```python
from build123d import *

# Parameters (mm, degrees)
F0_R          = 3
F0_R_2        = 2.5
F1_DEPTH      = 150
F2_R          = 2
F3_R          = 7
F6_DEPTH      = 30
F6_DEPTH_BACK = 30


# Not quite as in the source:
# - a feature names something its author has since deleted; it is built from what else it names


with BuildPart() as f1:
    # F0 (on Top) → F1 (new body)
    with BuildSketch(Plane.XY):
        with BuildLine():
            Line((18.15, -30), (30, -30))
            Line((30, -30), (30, -18.15))
            Line((30, -18.15), (27.5, -18.15))
            Line((27.5, -18.15), (27.5, -20.15))
            Line((27.5, -20.15), (21.5477069044, -20.15))
            ThreePointArc((21.5477069044, -20.15), (19.5, -15), (21.5477069044, -9.85))
            Line((21.5477069044, -9.85), (27.5, -9.85))
            Line((27.5, -9.85), (27.5, -11.85))
            Line((27.5, -11.85), (30, -11.85))
            Line((30, -11.85), (30, 11.85))
            Line((30, 11.85), (27.5, 11.85))
            Line((27.5, 11.85), (27.5, 9.85))
            Line((27.5, 9.85), (21.5477069044, 9.85))
            ThreePointArc((21.5477069044, 9.85), (19.5, 15), (21.5477069044, 20.15))
            Line((21.5477069044, 20.15), (27.5, 20.15))
            Line((27.5, 20.15), (27.5, 18.15))
            Line((27.5, 18.15), (30, 18.15))
            Line((30, 18.15), (30, 30))
            Line((30, 30), (18.15, 30))
            Line((18.15, 30), (18.15, 27.5))
            Line((18.15, 27.5), (20.15, 27.5))
            Line((20.15, 27.5), (20.15, 21.5477069044))
            ThreePointArc((20.15, 21.5477069044), (15, 19.5), (9.85, 21.5477069044))
            Line((9.85, 21.5477069044), (9.85, 27.5))
            Line((9.85, 27.5), (11.85, 27.5))
            Line((11.85, 27.5), (11.85, 30))
            Line((11.85, 30), (-11.85, 30))
            Line((-11.85, 30), (-11.85, 27.5))
            Line((-11.85, 27.5), (-9.85, 27.5))
            Line((-9.85, 27.5), (-9.85, 21.5477069044))
            ThreePointArc((-9.85, 21.5477069044), (-15, 19.5), (-20.15, 21.5477069044))
            Line((-20.15, 21.5477069044), (-20.15, 27.5))
            Line((-20.15, 27.5), (-18.15, 27.5))
            Line((-18.15, 27.5), (-18.15, 30))
            Line((-18.15, 30), (-30, 30))
            Line((-30, 30), (-30, 18.15))
            Line((-30, 18.15), (-27.5, 18.15))
            Line((-27.5, 18.15), (-27.5, 20.15))
            Line((-27.5, 20.15), (-21.5477069044, 20.15))
            ThreePointArc((-21.5477069044, 20.15), (-19.5, 15), (-21.5477069044, 9.85))
            Line((-21.5477069044, 9.85), (-27.5, 9.85))
            Line((-27.5, 9.85), (-27.5, 11.85))
            Line((-27.5, 11.85), (-30, 11.85))
            Line((-30, 11.85), (-30, -11.85))
            Line((-30, -11.85), (-27.5, -11.85))
            Line((-27.5, -11.85), (-27.5, -9.85))
            Line((-27.5, -9.85), (-21.5477069044, -9.85))
            ThreePointArc((-21.5477069044, -9.85), (-19.5, -15), (-21.5477069044, -20.15))
            Line((-21.5477069044, -20.15), (-27.5, -20.15))
            Line((-27.5, -20.15), (-27.5, -18.15))
            Line((-27.5, -18.15), (-30, -18.15))
            Line((-30, -18.15), (-30, -30))
            Line((-30, -30), (-18.15, -30))
            Line((-18.15, -30), (-18.15, -27.5))
            Line((-18.15, -27.5), (-20.15, -27.5))
            Line((-20.15, -27.5), (-20.15, -21.5477069044))
            ThreePointArc((-20.15, -21.5477069044), (-15, -19.5), (-9.85, -21.5477069044))
            Line((-9.85, -21.5477069044), (-9.85, -27.5))
            Line((-9.85, -27.5), (-11.85, -27.5))
            Line((-11.85, -27.5), (-11.85, -30))
            Line((-11.85, -30), (11.85, -30))
            Line((11.85, -30), (11.85, -27.5))
            Line((11.85, -27.5), (9.85, -27.5))
            Line((9.85, -27.5), (9.85, -21.5477069044))
            ThreePointArc((9.85, -21.5477069044), (15, -19.5), (20.15, -21.5477069044))
            Line((20.15, -21.5477069044), (20.15, -27.5))
            Line((20.15, -27.5), (18.15, -27.5))
            Line((18.15, -27.5), (18.15, -30))
        make_face()
        with Locations((-25, -25)):
            Circle(F0_R, mode=Mode.SUBTRACT)
        with Locations((-15, -15)):
            Circle(F0_R_2, mode=Mode.SUBTRACT)
        with Locations((25, -25)):
            Circle(F0_R, mode=Mode.SUBTRACT)
        with Locations((15, -15)):
            Circle(F0_R_2, mode=Mode.SUBTRACT)
        with Locations((-25, 25)):
            Circle(F0_R, mode=Mode.SUBTRACT)
        with Locations((-15, 15)):
            Circle(F0_R_2, mode=Mode.SUBTRACT)
        Polygon((-7, 22), (-7, 27.5), (0, 27.5), (7, 27.5), (7, 22), (10, 16), (10, 10), (16, 10), (22, 7), (27.5, 7), (27.5, 0), (27.5, -7), (22, -7), (16, -10), (10, -10), (10, -16), (7, -22), (7, -27.5), (0, -27.5), (-7, -27.5), (-7, -22), (-10, -16), (-10, -10), (-16, -10), (-22, -7), (-27.5, -7), (-27.5, 0), (-27.5, 7), (-22, 7), (-16, 10), (-10, 10), (-10, 16), align=None, mode=Mode.SUBTRACT)
        with Locations((15, 15)):
            Circle(F0_R_2, mode=Mode.SUBTRACT)
        with Locations((25, 25)):
            Circle(F0_R, mode=Mode.SUBTRACT)
    extrude(amount=F1_DEPTH)

    # F2
    f2_edges = [f1.edges().sort_by_distance(p)[0] for p in [
        (-7, 27.5, 75),
        (7, 27.5, 75),
    ]]
    fillet(f2_edges, radius=F2_R)

    # F3
    f3_edges = [f1.edges().sort_by_distance(p)[0] for p in [
        (-10, 16, 75),
        (10, 16, 75),
    ]]
    fillet(f3_edges, radius=F3_R)

    # F5 (on Right) → F6 (cut, two sides)
    with BuildSketch(Plane.YZ) as f6_sk:
        Polygon((14.9420964297, -75.7011932878), (30, 0), (-77.5301070084, 21.3890681496), (-92.5880105787, -54.3121251382), align=None)
        Polygon((89.181769874, 100.6332945306), (123.8334032044, 184.2897376752), (4.6516333304, 233.6564431446), (-30, 150), align=None)
    extrude(amount=F6_DEPTH, mode=Mode.SUBTRACT)
    extrude(f6_sk.sketch, amount=-F6_DEPTH_BACK, mode=Mode.SUBTRACT)


solid = f1.part
```
CAD build for the part. Positions are in the model's coordinates, mm. A direction names the side the tool comes from. Coordinates: 2 decimals unless noted, no trailing zeros. Order: outer loops, then holes, each group sorted by start corner. A loop starts at its lowest first (then second) coordinate and runs counter-clockwise, first axis right, second up. Notation, with made-up numbers: (72, 72.5) - (110, 72.5) arc R28 cw to (110, 90.5) - close; hole circle Ø1 at (83.5, 60). An arc over 180 degrees is marked (long way). Use a Markdown table: item, result. Add a question column.
(1) Saw through at B-B (y = -1). Give the cut face in (x, z), then the cut area to 3 significant figures.
(2) Flat gauge pins, fed straight in: pin 1 (10 mm diameter, centred on x = -9.5, y = -1.5, fed in from -Z); pin 2 (2 mm diameter, centred on y = 13.5, z = 118, fed in from +X); pin 3 (10 mm diameter, centred on x = 11.5, y = 9, fed in from -Z); pin 4 (8 mm diameter, centred on x = 15, y = -15, fed in from +Z). Where does each tip first touch, or does it go through?
(3) Saw through at D-D (z = 90.5). Count the separate pieces of the cut face and the enclosed holes in it, then the cut area to 3 significant figures.
(4) Saw through at C-C (x = -2.5). Give the cut face in (y, z), then the cut area to 3 significant figures.
(5) Which spindle directions (+Z, -Z, +X, -X, +Y, -Y) get a long thin tool onto all of the face, cutting with end or side? Do faces 3 (the face through (-24, 30, 62)), 4 (the face through (-19, 8.5, 68.4)). Say none if no direction does.
(6) Saw through at A-A (x = -25). Give the cut face in (y, z).
(7) Pull direction X, two halves, no side cores. Call faces 1 (the face through (11.25, 10.97, 133.03)), 2 (the face through (-25, -7, 73)): +X half, -X half, draft (parallel to the pull), parting line (faces both ways), or undercut.
(8) Drill centre lines: line 1 along X through (y, z) = (-25, 81.5); line 2 along X through (y, z) = (-15, 63). Where is each one in solid material? Low to high. Write a range as [from, to].
Solved:
| question | item | result |
|---|---|---|
| 1 | outline | (-30, 6.17) - (-27.5, 6.17) - (-27.5, 137.99) - (-30, 137.99) - close; (27.5, 6.17) - (30, 6.17) - (30, 137.99) - (27.5, 137.99) - close |
| 1 | area | 659 mm² |
| 2 | pin 1 | passes through |
| 2 | pin 2 | stops at x = 19.93 |
| 2 | pin 3 | stops at z = 3.18 |
| 2 | pin 4 | stops at z = 145.44 |
| 3 | separate pieces | 1 |
| 3 | enclosed holes | 9 |
| 3 | area | 1,080 mm² |
| 4 | outline | (-30, 11.93) - (-27.5, 11.44) - (-27.5, 148.96) - (-30, 150) - close; (27.5, 0.5) - (30, 0) - (30, 125.15) - (27.5, 126.18) - close |
| 4 | area | 658 mm² |
| 5 | face 3 | +Z, -Z, +X, -X, +Y |
| 5 | face 4 | +Z, -Z |
| 6 | outline | (-30, 11.93) - (-28, 11.54) - (-28, 149.17) - (-30, 150) - close; (-22, 10.34) - (-20.15, 9.98) - (-20.15, 145.92) - (-22, 146.69) - close; (-9.85, 7.93) - (-7, 7.36) - (-7, 140.47) - (-9.85, 141.65) - close; (7, 4.57) - (9.85, 4.01) - (9.85, 133.49) - (7, 134.67) - close; (20.15, 1.96) - (22, 1.59) - (22, 128.46) - (20.15, 129.23) - close; (28, 0.4) - (30, 0) - (30, 125.15) - (28, 125.98) - close |
| 7 | face 1 | draft |
| 7 | face 2 | undercut |
| 8 | line 1 | x = [-30, -28], [-22, -20.15], [-9.85, -7], [7, 9.85], [20.15, 22], [28, 30] |
| 8 | line 2 | x = [-19.5, -17.5], [-12.5, -10], [10, 12.5], [17.5, 19.5] |
